Geometry check sheet. Reference: the model listing, model coordinates, mm. A direction names the side the tool comes from. Give positions to 0.01 mm unless a question says otherwise; leave off trailing zeros. Order: outer loops, then holes, each group sorted by start corner. A loop starts at its lowest first (then second) coordinate and runs counter-clockwise, first axis right, second up. Notation, with made-up numbers: M -22,3 L 25,3 A25 cw 25,40 Z; hole C 67,7.25 d3. An arc over 180 degrees is marked long. Answer as a JSON object with one key per item and string values. Group by question number.
from build123d import *

# Parameters (mm, degrees)
F0_R     = 31.115
F1_DEPTH = 174
F2_SIZE2 = 8.1603840177
F2_SIZE  = 17.5
F3_R     = 12.5
F4_DEPTH = 3.5
F5_R     = 16.45
F6_DEPTH = 20.3
F7_R     = 11.8
F8_DEPTH = 25.4


with BuildPart() as f1:
    # F0 (on Top) → F1 (new body)
    with BuildSketch(Plane.XY):
        Circle(F0_R)
    extrude(amount=F1_DEPTH)

    # F2
    f2_edges = [f1.edges().sort_by_distance(p)[0] for p in [
        (-31.115, 0, 174),
    ]]
    f2_side = f1.faces().sort_by_distance((0, 0, 174))[0]
    chamfer(f2_edges, length=F2_SIZE, length2=F2_SIZE2, reference=f2_side)

    # F3 (on face) → F4 (join)
    with BuildSketch(Plane.XY.offset(174)):
        Circle(F3_R)
    extrude(amount=F4_DEPTH)

    # F5 (on face) → F6 (join)
    with BuildSketch(Plane.XY.offset(177.5)):
        Circle(F5_R)
    extrude(amount=F6_DEPTH)

    # F7 (on face) → F8 (join)
    with BuildSketch(Plane.XY.offset(197.8)):
        Circle(F7_R)
    extrude(amount=F8_DEPTH)


solid = f1.part
1. Access from +Z, -Z, +X, -X, +Y, -Y to the whole of each face (thin tool, end or side, straight path). Record for faces 1 (the flat face through (12.04, -3.97, 174)), 2 (the flat face through (0, 0, 223.2)), 3 (the cylindrical face through (-3.566, -16.059, 187.508)).
2. Cross-section at C-C (z = 112.5). Record the cut outline in (x, y) (3 decimals).
3. Release check for a two-part mould opening along Z. For faces 4 (the flat face through (0, 0, 0)), 5 (the flat face through (3.6, 12.3, 177.5)), 6 (the flat face through (7, -11, 197.8)) record: released by +Z, released by -Z, zero draft, split by the parting line, or undercut.
4. Thickness scan on line 1 along X through (y, z) = (1.5, 20); line 2 along Z through (x, y) = (-8, -11.5); line 3 along X through (y, z) = (-10.5, 41). Record the ranges inside material, lowest first. Write a range as [from, to].
5. Cross-section at A-A (y = 0). Record the cut outline in (x, z) (3 decimals).
6. Depth check by flat-ended pin: pin 1 (12 mm diameter, centred on x = -5, z = 83.5, fed in from -Y) (3 decimals); pin 2 (1 mm diameter, centred on y = 25, z = 150.5, fed in from +X); pin 3 (3 mm diameter, centred on x = 7.5, z = 58, fed in from +Y). Enter the tip coordinate at first touch or a pass-through.
Report:
{
 "1": {"face 1": "none", "face 2": "+Z, +X, -X, +Y, -Y", "face 3": "+Z"},
 "2": {"outline": "C 0,0 d62.23"},
 "3": {"face 4": "released by -Z", "face 5": "undercut", "face 6": "released by +Z"},
 "4": {"line 1": "x = [-31.08, 31.08]", "line 2": "z = [0, 173.82], [177.5, 197.8]", "line 3": "x = [-29.29, 29.29]"},
 "5": {"outline": "M -31.115,0 L 31.115,0 L 31.115,165.84 L 13.615,174 L 12.5,174 L 12.5,177.5 L 16.45,177.5 L 16.45,197.8 L 11.8,197.8 L 11.8,223.2 L -11.8,223.2 L -11.8,197.8 L -16.45,197.8 L -16.45,177.5 L -12.5,177.5 L -12.5,174 L -13.615,174 L -31.115,165.84 Z"},
 "6": {"pin 1": "stops at y = -31.115", "pin 2": "stops at x = 19.18", "pin 3": "stops at y = 30.53"}
}
